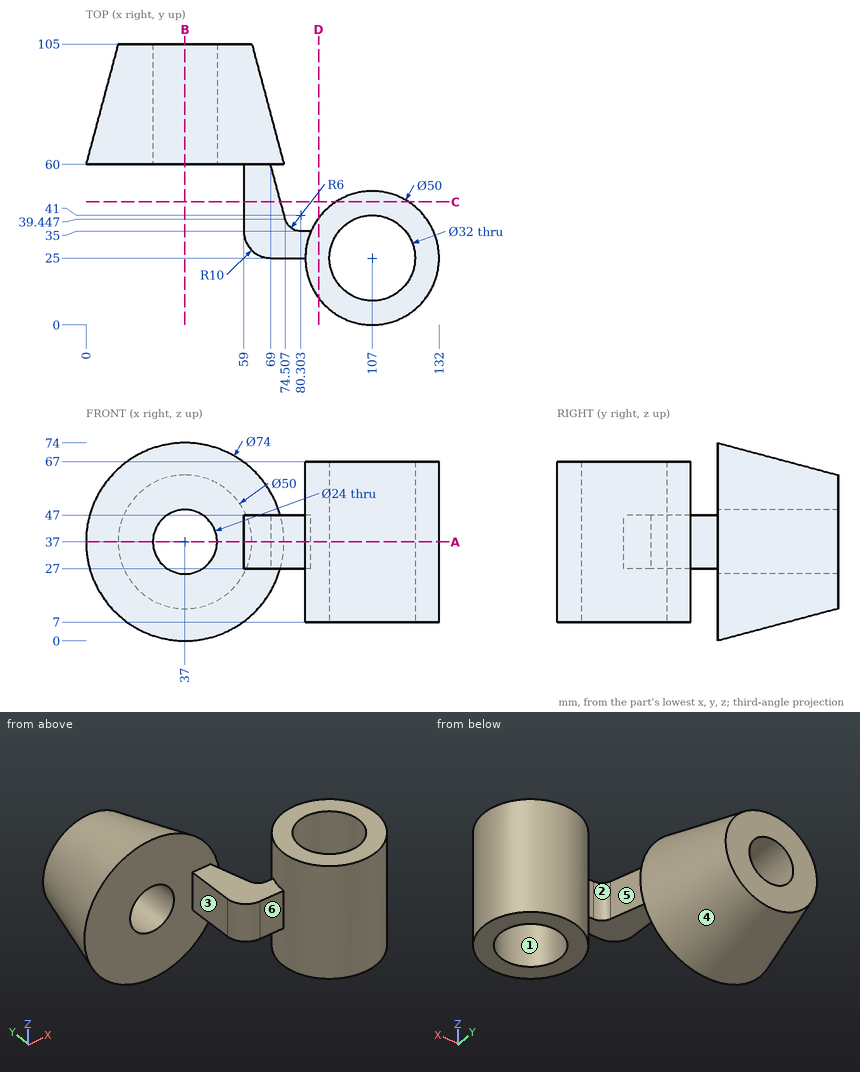
Geometry check sheet. Reference: drawing and pictorial views, mm from the part's lowest x, y, z. A direction names the side the tool comes from. Coordinates: 2 decimals unless noted, no trailing zeros. Order: outer loops, then holes, each group sorted by start corner. A loop starts at its lowest first (then second) coordinate and runs counter-clockwise, first axis right, second up.
Item 1: Tool access check on the marked faces 1, 2 and 3. Record the directions out of +Z, -Z, +X, -X, +Y, -Y that give a thin tool (end or side, any length) a straight path to the whole face; none if there is none.
Item 2: Section check D-D (x = 87). Enter the section's corners in (y, z).
Item 3: Section check B-B (x = 37). Enter the section's corners in (y, z).
Item 4: Section check C-C (y = 46). Enter the section's corners in (x, z) (1 decimal), plus the area to 3 significant figures.
Item 5: Section check A-A (z = 37). Enter the section's corners in (x, y).
Item 6: Mould release check, pull along X, two halves, no side actions. Record for the marked faces 4, 5 and 6: released by +X, released by -X, zero draft, split by the parting line, or undercut.
Item 7: Scan lines: line 1 along Y through (x, z) = (107, 31.5); line 2 along Y through (x, z) = (21.5, 19); line 3 along X through (y, z) = (19, 20). Record each from-to range of solid material in increasing order.
Item 8: Depth check by flat-ended pin: pin 1 (6 mm diameter, centred on x = 66, y = 42, fed in from -Z); pin 2 (20 mm diameter, centred on x = 67, y = 48, fed in from +Z); pin 3 (6 mm diameter, centred on y = 47, z = 36.5, fed in from -X). Enter the tip coordinate at first touch or a pass-through.
Check sheet entries:
1. face 1: +Z, -Z
1. face 2: +Z, -Z, +Y
1. face 3: +Z, -Z, -X, -Y
2. outline: (10, 7) - (40, 7) - (40, 67) - (10, 67) - close
3. outline: (60, 0) - (105, 12) - (105, 25) - (60, 25) - close; (60, 49) - (105, 49) - (105, 62) - (60, 74) - close
4. outline: (59, 27) - (72.8, 27) - (72.8, 47) - (59, 47) - close; (93.4, 7) - (120.6, 7) - (120.6, 67) - (93.4, 67) - close
4. area: 1,900 mm2
5. outline: (0, 60) - (25, 60) - (25, 105) - (12, 105) - close; (49, 60) - (59, 60) - (59, 35) arc R10 ccw to (69, 25) - (82, 25) arc R25 ccw (long way) to (84.09, 35) - (80.3, 35) arc R6 cw to (74.51, 39.45) - (69, 60) - (74, 60) - (62, 105) - (49, 105) - close; hole circle Ø32 at (107, 25)
6. face 4: split by the parting line
6. face 5: undercut
6. face 6: zero draft
7. line 1: y = 0 to 9, 41 to 50
7. line 2: y = 60 to 105
7. line 3: x = 82.73 to 92.17, 121.83 to 131.27
8. pin 1: stops at z = 27
8. pin 2: stops at z = 47
8. pin 3: stops at x = 59
